Read the model definition and answer for the solid it produces. Units are mm, in the model's axes. Face numbers are marked on the shaded views. A direction names the side the tool comes from. Coordinates: 2 decimals unless noted, no trailing zeros. Order: outer loops, then holes, each group sorted by start corner. A loop starts at its lowest first (then second) coordinate and runs counter-clockwise, first axis right, second up.
Autodesk Inventor part; units mm, degrees
ref_plane "YZ Plane" through (0, 0, 0) normal (1, 0, 0) x (0, 1, 0)
ref_plane "XZ Plane" through (0, 0, 0) normal (0, 1, 0) x (-1, 0, 0)
ref_plane "XY Plane" through (0, 0, 0) normal (0, 0, 1) x (1, 0, 0)
sketch "Sketch1" plane through (0, 0, 0) normal (0, 0, 1) x (1, 0, 0)
  arc A0 (7.5, 0) -> (-7.5, 0) centre (0, 0) ccw
  line L0 (-7.5, 0) -> (7.5, 0)
  dimension "d2" = 7.5
revolve "Revolution1" add sketch "Sketch1" angle 180 mid plane about axis through (-7.5, 0, 0) along (1, 0, 0)
sketch "Sketch2" plane through (0, 0, 0) normal (1, 0, 0) x (0, 1, 0)
  line L0 (24.4009, -6.216) -> (37.3287, -2.2636)
  line L1 (33.5279, 10.1684) -> (20.6001, 6.216)
  arc A0 (20.6001, 6.216) -> (24.4009, -6.216) centre (28.4534, 1.82) ccw
  arc A1 (33.5279, 10.1684) -> (11.2086, 9.8739) centre (22.5005, 0) ccw
  arc A2 (11.6815, -10.3899) -> (37.3287, -2.2636) centre (22.5005, 0) ccw
  arc A3 (11.6815, -10.3899) -> (0, -6.4952) centre (-1.1685, -29.4655) ccw
  arc A4 (0, 6.4952) -> (11.2086, 9.8739) centre (-0.8152, 29.4807) ccw
  line L2 (0, -6.4952) -> (0, 6.4952)
  line L3 (0, 7.5) -> (0, -7.5)
  point P0 (0, 0)
  dimension "d15" = 23
  dimension "d16" = 23
extrude "Extrusion1" add sketch "Sketch2" along normal mid plane 7.5
properties part number "Spanner"
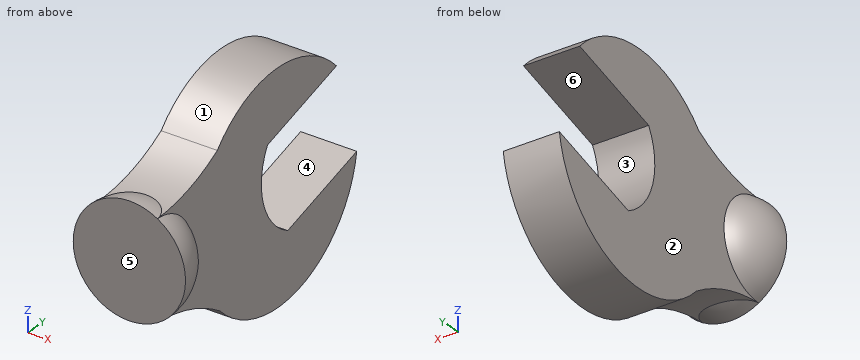
1) Straight lines are drawn through the part: line 1 (X direction, y = 19, z = -3); line 2 (Y direction, x = -0.5, z = 1.5); line 3 (Z direction, x = 3, y = 29). For each, find the intervals that lie inside material, in ascending order.
A:
line 1: x = -3.75 to 3.75
line 2: y = 0 to 19.46
line 3: z = -13.52 to -4.81, 8.78 to 13.52
2) Which of the six approach directions +Z, -Z, +X, -X, +Y, -Y give full straight-line access (tool end or side, diameter ignored) to the marked faces 5 and 6?
A:
face 5: +Z, -Z, +X, -X, -Y
face 6: +X, -X, +Y
3) A cutting plane is placed at B-B, the plane y = 32. Determine the outline of the cut face in (x, z).
A:
outline: (-3.75, -11.61) - (3.75, -11.61) - (3.75, -3.89) - (-3.75, -3.89) - close; (-3.75, 9.7) - (3.75, 9.7) - (3.75, 11.61) - (-3.75, 11.61) - close
4) A cutting plane is placed at A-A, the plane z = -5.5. Determine the outline of the cut face in (x, y), and give its area (3 significant figures).
A:
outline: (-5.1, 0) - (5.1, 0) arc R5.1 ccw to (3.75, 3.46) - (3.75, 23.22) - (-3.75, 23.22) - (-3.75, 3.46) arc R5.1 ccw to start; (-3.75, 26.74) - (3.75, 26.74) - (3.75, 36.46) - (-3.75, 36.46) - close
area: 253 mm2
5) Flat-ended cylindrical pins translate along their axes: pin 1 Ø15 at (y, z) = (25.5, 5) entering from +X; pin 2 Ø6 at (x, y) = (4.5, 22.5) entering from -Z; pin 3 Ø1 at (x, y) = (0.5, 20) entering from +Z; pin 4 Ø4 at (y, z) = (22.5, 6.5) entering from -X. Find the tip coordinate at first contact, or state that the pin passes through.
A:
pin 1: stops at x = 3.75
pin 2: stops at z = -15
pin 3: stops at z = 14.87
pin 4: stops at x = -3.75
6) A cutting plane is placed at D-D, the plane y = 25. Determine the outline of the cut face in (x, z), and give its area (3 significant figures).
A:
outline: (-3.75, -14.79) - (3.75, -14.79) - (3.75, -6.03) - (-3.75, -6.03) - close; (-3.75, 7.56) - (3.75, 7.56) - (3.75, 14.79) - (-3.75, 14.79) - close
area: 120 mm2
7) Determine the mould class of the marked faces 1, 2, 3 and 4 for opening direction Z: pulls with the +Z half, pulls with the -Z half, needs draft (parallel to the pull), parting line crosses it, or undercut.
A:
face 1: pulls with the +Z half
face 2: needs draft
face 3: undercut
face 4: undercut
8) A cutting plane is placed at C-C, the plane x = -0.75. Determine the outline of the cut face in (y, z), and give its area (3 significant figures).
A:
outline: (0, -7.46) arc R7.46 ccw to (2.98, -6.84) arc R23 cw to (11.68, -10.39) arc R15 ccw to (37.33, -2.26) - (24.4, -6.22) arc R9 cw to (20.6, 6.22) - (33.53, 10.17) arc R15 ccw to (11.21, 9.87) arc R23 cw to (3.05, 6.81) arc R7.46 ccw to (0, 7.46) - close
area: 620 mm2
